Autodesk Inventor part; units mm, degrees
ref_plane "YZ Plane" through (0, 0, 0) normal (1, 0, 0) x (0, 1, 0)
ref_plane "XZ Plane" through (0, 0, 0) normal (0, 1, 0) x (-1, 0, 0)
ref_plane "XY Plane" through (0, 0, 0) normal (0, 0, 1) x (1, 0, 0)
sketch "Sketch1" plane through (0, 0, 0) normal (0, 0, 1) x (1, 0, 0)
  line L0 (0, 0) -> (28.575, 0)
  line L1 (28.575, 0) -> (28.575, 203.2)
  line L2 (28.575, 203.2) -> (0, 203.2)
  line L3 (0, 203.2) -> (0, 0)
  line L4 (31.75, 209.55) -> (31.75, 0)
  line L5 (-3.175, 0) -> (-3.175, 209.55)
  line L6 (-3.175, 209.55) -> (31.75, 209.55)
  line L7 (-3.175, 0) -> (31.75, 0)
  dimension "d0" = 28.575
  dimension "d1" = 203.2
  dimension "d2" = 3.175
  dimension "d24" = 6.35
  dimension "d25" = 3.175
extrude "Extrusion1" add sketch "Sketch1" along normal blind 28.575 contours L7 L5 L6 L4 L1 L2 L3
sketch "Sketch2" plane through (31.75, 0, 0) normal (1, 0, 0) x (0, 0, -1)
  line L0 (0, 0) -> (-28.575, 0)
  line L1 (0, 209.55) -> (0, 0)
  point P0 (-23.8125, 5.207)
  point P1 (-4.7625, 5.207)
  dimension "d5" = 5.207
  dimension "d6" = 19.05
  dimension "d7" = 28.575
  dimension "d8" = 4.7625
hole "Hole1" at (31.75, 5.207, 23.8125) at (31.75, 5.207, 4.7625) direction (-1, 0, 0) diameter 5.1054 end through all
sketch "Sketch4" plane through (31.75, 0, 0) normal (1, 0, 0) x (0, 0, -1)
  line L0 (-28.575, 0) -> (-28.575, 209.55)
  line L1 (0, 209.55) -> (0, 0)
  point P0 (-23.495, 206.2387)
  point P1 (-5.08, 206.2387)
  dimension "d26" = 5.08
  dimension "d27" = 5.08
  dimension "d28" = 18.415
hole "Hole3" at (31.75, 206.2387, 23.495) at (31.75, 206.2387, 5.08) direction (-1, 0, 0) diameter 5.08 depth 10.9728 tip angle 118
properties material "Aluminum 6061"
Design review of the part built by this model. Coordinates are the model's own, in mm. A direction names the side the tool comes from. Give positions to 0.01 mm unless a question says otherwise; leave off trailing zeros. Loops run counter-clockwise (first coordinate to the right, second up) from the corner with the lowest first, then second, coordinate; pieces in that order, holes last. Notation, with made-up numbers: (20, -32.75) -> (72, -32.75) arc R31 ccw to (72, -3.75) -> close; hole circle Ø1 at (80.5, -14.5). An arc over 180 degrees is marked (long way). Write each question's results on one line, items separated by ' | '.
Q1. Machinability: for faces 5 (the face through (28.575, 100, 14)), 6 (the face through (26.19, 203.72, 5.41)), 7 (the face through (-1.61, 3.48, 6.64)), which of the approach directions +Z, -Z, +X, -X, +Y, -Y give a long, thin tool a straight path to every point of the face, cutting with its end or side? Answer none if there is none.
Reply:
face 5: +Z, -Z, -Y | face 6: +X | face 7: +X, -X
Q2. The part is to be moulded in two halves that separate along Y. For faces 1 (the face through (-1.61, 6.185, 21.454)), 2 (the face through (14, 203.2, 14)), 3 (the face through (26.19, 203.72, 23.83)), 4 (the face through (31.75, 106, 14)), say which applies: +Y half, -Y half, draft (parallel to the pull), parting line (faces both ways), or undercut.
Reply:
face 1: undercut | face 2: -Y half | face 3: undercut | face 4: draft
Q3. Take a section at A-A, the plane y = 55. Write out the cut boundary in (x, z) (3 decimals).
Reply:
outline: (-3.175, 0) -> (0, 0) -> (0, 28.575) -> (-3.175, 28.575) -> close; (28.575, 0) -> (31.75, 0) -> (31.75, 28.575) -> (28.575, 28.575) -> close
Q4. For pin 1 Ø1 at (x, z) = (12, 21) entering from -Y; pin 2 Ø3 at (y, z) = (5.21, 23.81) entering from +X, all flat-tipped, find the tip position at first contact; note any pin that passes through.
Reply:
pin 1: stops at y = 203.2 | pin 2: passes through
Q5. Wall thickness on L1, parallel to X at y = 54.5, z = 11.25 (3 decimals); L2, parallel to Y at x = 24.75, z = 5.08; L3, parallel to Y at x = 10, z = 20.75: over which ranges is each line inside the solid? List them lowest first.
Reply:
L1: x = -3.175 to 0, 28.575 to 31.75 | L2: y = 203.2 to 203.7, 208.78 to 209.55 | L3: y = 203.2 to 209.55
Q6. Take a section at B-B, the plane x = 11.5. Write out the cut boundary in (y, z) (3 decimals).
Reply:
outline: (203.2, 0) -> (209.55, 0) -> (209.55, 28.575) -> (203.2, 28.575) -> close
Q7. Take a section at C-C, the plane x = 23. Write out the cut boundary in (y, z) (3 decimals).
Reply:
outline: (203.2, 0) -> (209.55, 0) -> (209.55, 28.575) -> (203.2, 28.575) -> close; hole circle Ø5.08 at (206.239, 5.08); hole circle Ø5.08 at (206.239, 23.495)
